Verification items for this drawing (mm, ordinates from the low corner). A direction names the side the tool comes from. Give positions to 0.01 mm unless a question says otherwise; leave off trailing zeros. Loops run counter-clockwise (first coordinate to the right, second up) from the corner with the lowest first, then second, coordinate; pieces in that order, holes last. Notation, with made-up numbers: M -33,24.5 L 23,24.5 A18 ccw 23,40.5 Z; hole C -1,-36 d5. An arc over 180 degrees is marked long. Put each result on its own line as item: value. Start each with the question number.
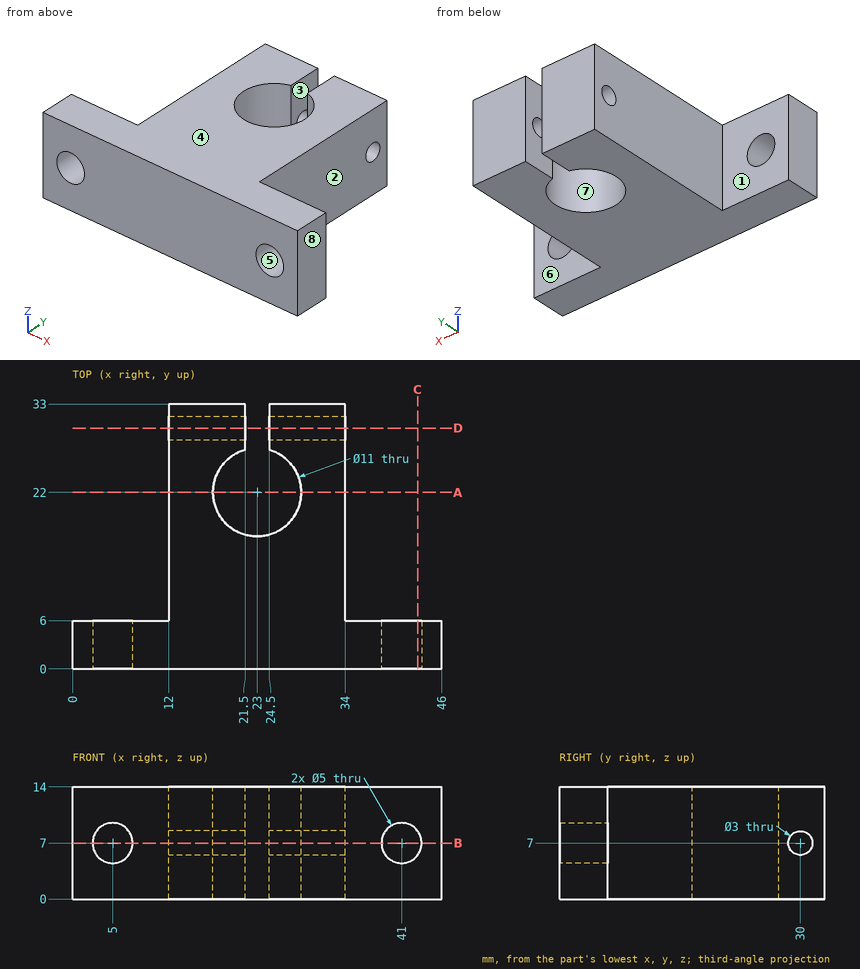
Q1. Release check for a two-part mould opening along X. For the marked faces 6, 7 and 8 record: pulls with the +X half, pulls with the -X half, needs draft (parallel to the pull), parting line crosses it, or undercut.
Q2. Cross-section at A-A, the plane y = 22. Record the boundary of the cut face in (x, z).
Q3. Cross-section at D-D, the plane y = 30. Record the boundary of the cut face in (x, z).
Q4. Go/stop test with flat-tipped pins: pin 1 (2.5 mm diameter, centred on y = 30, z = 7, fed in from +X); pin 2 (3.5 mm diameter, centred on x = 6.5, z = 10, fed in from +Y); pin 3 (1.7 mm diameter, centred on y = 29, z = 9, fed in from +X); pin 4 (6 mm diameter, centred on y = 11.5, z = 8.5, fed in from -X). Record where each tip stops, or that it passes through.
Q5. Set-up check for the marked faces 1, 2, 3, 4 and 5: record each of +Z, -Z, +X, -X, +Y, -Y from which the full face is reachable in a straight line by a thin tool's end or side.
Q6. Scan lines: L1, parallel to Z at x = 5, y = 1; L2, parallel to Y at x = 28, z = 7; L3, parallel to Y at x = 3.5, z = 1.5. Record each from-to range of solid material in increasing order.
Q7. Cross-section at C-C, the plane x = 43. Record the boundary of the cut face in (y, z), then the cut area to 3 significant figures.
Q8. Cross-section at B-B, the plane z = 7. Record the boundary of the cut face in (x, y).
Ans:
1. face 6: needs draft
1. face 7: undercut
1. face 8: pulls with the +X half
2. outline: M 12,0 L 17.5,0 L 17.5,14 L 12,14 Z; M 28.5,0 L 34,0 L 34,14 L 28.5,14 Z
3. outline: M 12,0 L 21.5,0 L 21.5,5.5 L 12,5.5 Z; M 12,8.5 L 21.5,8.5 L 21.5,14 L 12,14 Z; M 24.5,0 L 34,0 L 34,5.5 L 24.5,5.5 Z; M 24.5,8.5 L 34,8.5 L 34,14 L 24.5,14 Z
4. pin 1: passes through
4. pin 2: stops at y = 6
4. pin 3: stops at x = 34
4. pin 4: stops at x = 12
5. face 1: +Z, -Z, -X, +Y
5. face 2: +Z, -Z, +X, +Y
5. face 3: +Z, -Z, +Y
5. face 4: +Z, +X, -X, +Y, -Y
5. face 5: +Y, -Y
6. L1: z = 0 to 4.5, 9.5 to 14
6. L2: y = 0 to 19.71, 24.29 to 28.5, 31.5 to 33
6. L3: y = 0 to 6
7. outline: M 0,0 L 6,0 L 6,5.5 L 0,5.5 Z; M 0,8.5 L 6,8.5 L 6,14 L 0,14 Z
7. area: 66.0 mm^2
8. outline: M 0,0 L 2.5,0 L 2.5,6 L 0,6 Z; M 7.5,0 L 38.5,0 L 38.5,6 L 34,6 L 34,28.5 L 24.5,28.5 L 24.5,27.29 A5.5 cw long 21.5,27.29 L 21.5,28.5 L 12,28.5 L 12,6 L 7.5,6 Z; M 12,31.5 L 21.5,31.5 L 21.5,33 L 12,33 Z; M 24.5,31.5 L 34,31.5 L 34,33 L 24.5,33 Z; M 43.5,0 L 46,0 L 46,6 L 43.5,6 Z
